Geometry: final body of the model. Coordinates: model frame, mm. Face numbers are marked on the shaded views. Round coordinates to 2 decimals unless told otherwise and drop trailing zeros. Order: outer loops, then holes, each group sorted by start corner. A loop starts at its lowest first (then second) coordinate and runs counter-clockwise, first axis right, second up. Notation, with made-up numbers: M -14,5 L -2,5 A16 cw -2,13 Z; hole C 27.5,24.5 d10. An arc over 180 degrees is marked long. Put each result on its own line as item: value. Start each with the question number.
1) Material intervals for probe 1 along X at (y, z) = (3, 5.25); probe 2 along Y at (x, z) = (42.5, 6); probe 3 along X at (y, z) = (16, 6.75), sorted ascending. Write a range as [from, to].
2) First-contact query: P1, Ø2, axis at y = -26, z = 3, coming from the -X side; P2, Ø2.5, axis at x = 0.5, y = -51, coming from the +Z side; P3, Ø2, axis at x = -36.5, z = 3.5, coming from the +Y side. Flat tips, straight axial feed; report the tip coordinate or a pass-through.
3) Section B-B, the plane y = -21. Return loops of the section in (x, z), then the cut area to 3 significant figures.
4) Section D-D, the plane y = 10. Return loops of the section in (x, z).
5) Section C-C, the plane z = 6.75. Count the separate pieces of the cut face and the enclosed holes in it, then the cut area to 3 significant figures.
6) Draft query along X for the marked faces 1, 2 and 3. Return one class per face: pulls with the +X half, pulls with the -X half, needs draft (parallel to the pull), parting line crosses it, or undercut.
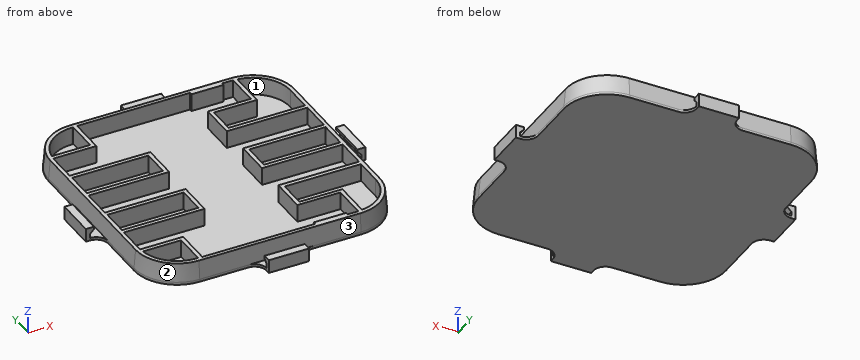
from build123d import *

# Parameters (mm, degrees)
F4_DEPTH     = 1.4
F5_W         = 30
F5_H         = 13.3
F5_W_2       = 12
F5_H_2       = 1
F6_DEPTH     = 6.6
F8_DEPTH     = 6.6
F9_W         = 14
F9_H         = 13.5
F10_DEPTH    = 6.6
F11_W        = 28.3875793553
F11_H        = 10.3
F12_DEPTH    = 6.6
F14_DEPTH    = 5.001
F15_T1_DEPTH = 1


# Not quite as in the source:
# - a fillet or chamfer that OpenCascade refuses, or shapes differently, is made with other operations: its cross-section is extruded or revolved along the edge and cut away or added


with BuildPart() as f2:
    # F2: sweep along a path in F0
    with BuildLine(Plane.XY) as f2_path:
        ThreePointArc((52, 30), (45.5563491861, 45.5563491861), (30, 52))
        Line((30, 52), (0, 52))
        Line((0, 52), (-30, 52))
        ThreePointArc((-30, 52), (-45.5563491861, 45.5563491861), (-52, 30))
        Line((-52, 30), (-52, 0))
        Line((-52, 0), (-52, -30))
        ThreePointArc((-52, -30), (-45.5563491861, -45.5563491861), (-30, -52))
        Line((-30, -52), (0, -52))
        Line((0, -52), (30, -52))
        ThreePointArc((30, -52), (45.5563491861, -45.5563491861), (52, -30))
        Line((52, -30), (52, 0))
        Line((52, 0), (52, 30))
    # F1 (on Front) → F2 (sweep)
    with BuildSketch(Plane.XZ):
        Polygon((44, 8), (44, 0), (52, 0), (52, 1), (52, 5), (49, 5), (49, 4), (50.5, 2.5), (50.5, 1), (46, 1), (45.3875793553, 8), align=None)
    sweep(path=f2_path.line)

    # F3 (on Top) → F4 (join)
    with BuildSketch(Plane.XY):
        with BuildLine():
            ThreePointArc((-44, -30), (-39.8994949366, -39.8994949366), (-30, -44))
            Line((-30, -44), (30, -44))
            ThreePointArc((30, -44), (39.8994949366, -39.8994949366), (44, -30))
            Line((44, -30), (44, 30))
            ThreePointArc((44, 30), (39.8994949366, 39.8994949366), (30, 44))
            Line((30, 44), (-30, 44))
            ThreePointArc((-30, 44), (-39.8994949366, 39.8994949366), (-44, 30))
            Line((-44, 30), (-44, -30))
        make_face()
    extrude(amount=F4_DEPTH)

    # F5 (on face) → F6 (join, through all)
    with BuildSketch(Plane.XY.offset(1.4)):
        with Locations((29, 24.85)):
            Rectangle(F5_W, F5_H)
        with Locations((20, 43.5)):
            Rectangle(F5_W_2, F5_H_2)
        with Locations((29, 0.05)):
            Rectangle(F5_W, F5_H)
        with Locations((29, -24.75)):
            Rectangle(F5_W, F5_H)
        with Locations((20, -43.5)):
            Rectangle(F5_W_2, F5_H_2)
        with BuildLine():
            ThreePointArc((-30, 44), (-39.7211110476, 40.0747208398), (-43.9910685796, 30.5))
            Line((-43.9910685796, 30.5), (-14, 30.5))
            Line((-14, 30.5), (-14, 44))
            Line((-14, 44), (-30, 44))
        make_face()
        with BuildLine():
            Line((-43.9910685796, 30.5), (-44, 30.5))
            Line((-44, 30.5), (-44, 30))
            ThreePointArc((-44, 30), (-43.9977669668, 30.250039882), (-43.9910685796, 30.5))
        make_face()
        with BuildLine():
            Line((-44, -30.5), (-43.9910685796, -30.5))
            ThreePointArc((-43.9910685796, -30.5), (-43.9977669668, -30.250039882), (-44, -30))
            Line((-44, -30), (-44, -30.5))
        make_face()
        with BuildLine():
            Line((-30, -44), (-14, -44))
            Line((-14, -44), (-14, -30.5))
            Line((-14, -30.5), (-43.9910685796, -30.5))
            ThreePointArc((-43.9910685796, -30.5), (-39.7211110476, -40.0747208398), (-30, -44))
        make_face()
        with Locations((-29, 12.35)):
            Rectangle(F5_W, F5_H)
        with Locations((-29, -12.45)):
            Rectangle(F5_W, F5_H)
    extrude(amount=F6_DEPTH)

    # F7 (on face) → F8 (join, through all)
    with BuildSketch(Plane.XY.offset(1.4)):
        with BuildLine():
            Line((43.9298241195, -31.4), (30, -31.4))
            Line((30, -31.4), (30, -44))
            ThreePointArc((30, -44), (39.3914855055, -40.3826778819), (43.9298241195, -31.4))
        make_face()
        with BuildLine():
            ThreePointArc((43.9194109071, 31.5), (39.3541434669, 40.416333328), (30, 44))
            Line((30, 44), (30, 31.5))
            Line((30, 31.5), (43.9194109071, 31.5))
        make_face()
    extrude(amount=F8_DEPTH)

    # F9 (on face) → F10 (cut, through all)
    with BuildSketch(Plane.XY.offset(8)):
        with Locations((-21, 37.25)):
            Rectangle(F9_W, F9_H)
        with Locations((-21, -37.25)):
            Rectangle(F9_W, F9_H)
    extrude(amount=-F10_DEPTH, mode=Mode.SUBTRACT)

    # F11 (on face) → F12 (cut, through all)
    with BuildSketch(Plane.XY.offset(8)):
        with BuildLine():
            Line((-43.7428112244, 32), (-29.5, 32))
            Line((-29.5, 32), (-29.5, 43.8875793553))
            Line((-29.5, 43.8875793553), (-30, 43.8875793553))
            ThreePointArc((-30, 43.8875793553), (-39.0854196832, 40.5033332581), (-43.7428112244, 32))
        make_face()
        with BuildLine():
            Line((15.5, 19.6999999465), (43.8875793553, 19.6999999465))
            Line((43.8875793553, 19.6999999465), (43.8875793553, 29.9999999465))
            ThreePointArc((43.8875793553, 30), (40.3367361721, 39.274521317), (31.5, 43.8063340663))
            Line((31.5, 43.8063340663), (31.5, 29.9999999465))
            Line((31.5, 29.9999999465), (15.5, 29.9999999465))
            Line((15.5, 29.9999999465), (15.5, 19.6999999465))
        make_face()
        with Locations((29.6937896777, 0.05)):
            Rectangle(F11_W, F11_H)
        with BuildLine():
            Line((31.5, -29.9999999465), (31.5, -43.8063340663))
            ThreePointArc((31.5, -43.8063340663), (40.3367361721, -39.274521317), (43.8875793553, -30))
            Line((43.8875793553, -29.9999999465), (43.8875793553, -29.9))
            Line((43.8875793553, -29.9), (43.8875793553, -19.6999999465))
            Line((43.8875793553, -19.6999999465), (15.5, -19.6999999465))
            Line((15.5, -19.6999999465), (15.5, -29.9))
            Line((15.5, -29.9), (15.5, -29.9999999465))
            Line((15.5, -29.9999999465), (31.5, -29.9999999465))
        make_face()
        with Locations((-29.6937896777, 12.35)):
            Rectangle(F11_W, F11_H)
        with Locations((-29.6937896777, -12.45)):
            Rectangle(F11_W, F11_H)
        with BuildLine():
            Line((-29.5, -32), (-43.7428112244, -32))
            ThreePointArc((-43.7428112244, -32), (-39.0854196832, -40.5033332581), (-30, -43.8875793553))
            Line((-30, -43.8875793553), (-29.5, -43.8875793553))
            Line((-29.5, -43.8875793553), (-29.5, -32))
        make_face()
    extrude(amount=-F12_DEPTH, mode=Mode.SUBTRACT)

    # F13 (on Top) → F14 (cut, through all)
    with BuildSketch(Plane.XY):
        with BuildLine():
            Line((52, -30), (52, -7.5))
            Line((52, -7.5), (46, -7.5))
            Line((46, -7.5), (46, -30))
            ThreePointArc((46, -30), (41.313708499, -41.313708499), (30, -46))
            Line((30, -46), (7.5, -46))
            Line((7.5, -46), (7.5, -52))
            Line((7.5, -52), (30, -52))
            ThreePointArc((30, -52), (45.5563491861, -45.5563491861), (52, -30))
        make_face()
        with BuildLine():
            Line((-30, -52), (-7.5, -52))
            Line((-7.5, -52), (-7.5, -46))
            Line((-7.5, -46), (-30, -46))
            ThreePointArc((-30, -46), (-41.313708499, -41.313708499), (-46, -30))
            Line((-46, -30), (-46, -7.5))
            Line((-46, -7.5), (-52, -7.5))
            Line((-52, -7.5), (-52, -30))
            ThreePointArc((-52, -30), (-45.5563491861, -45.5563491861), (-30, -52))
        make_face()
        with BuildLine():
            Line((-7.5, 46), (-7.5, 52))
            Line((-7.5, 52), (-30, 52))
            ThreePointArc((-30, 52), (-45.5563491861, 45.5563491861), (-52, 30))
            Line((-52, 30), (-52, 7.5))
            Line((-52, 7.5), (-46, 7.5))
            Line((-46, 7.5), (-46, 30))
            ThreePointArc((-46, 30), (-41.313708499, 41.313708499), (-30, 46))
            Line((-30, 46), (-7.5, 46))
        make_face()
        with BuildLine():
            ThreePointArc((30, 46), (41.313708499, 41.313708499), (46, 30))
            Line((46, 30), (46, 7.5))
            Line((46, 7.5), (52, 7.5))
            Line((52, 7.5), (52, 30))
            ThreePointArc((52, 30), (45.5563491861, 45.5563491861), (30, 52))
            Line((30, 52), (7.5, 52))
            Line((7.5, 52), (7.5, 46))
            Line((7.5, 46), (30, 46))
        make_face()
    extrude(amount=F14_DEPTH, mode=Mode.SUBTRACT)

    # F15: fillet of radius 4.5 on 8 edges, made by hand

    # F15_s2 → F15_t1 (join)
    with BuildSketch(Plane.XY):
        with BuildLine():
            ThreePointArc((-46, 12), (-47.3180194847, 8.8180194847), (-50.5, 7.5))
            Line((-50.5, 7.5), (-46, 7.5))
            Line((-46, 7.5), (-46, 12))
        make_face()
        with BuildLine():
            ThreePointArc((-12, 46), (-8.8180194847, 47.3180194847), (-7.5, 50.5))
            Line((-7.5, 50.5), (-7.5, 46))
            Line((-7.5, 46), (-12, 46))
        make_face()
        with BuildLine():
            ThreePointArc((12, 46), (8.8180194847, 47.3180194847), (7.5, 50.5))
            Line((7.5, 50.5), (7.5, 46))
            Line((7.5, 46), (12, 46))
        make_face()
        with BuildLine():
            ThreePointArc((12, -46), (8.8180194847, -47.3180194847), (7.5, -50.5))
            Line((7.5, -50.5), (7.5, -46))
            Line((7.5, -46), (12, -46))
        make_face()
        with BuildLine():
            ThreePointArc((-12, -46), (-8.8180194847, -47.3180194847), (-7.5, -50.5))
            Line((-7.5, -50.5), (-7.5, -46))
            Line((-7.5, -46), (-12, -46))
        make_face()
        with BuildLine():
            ThreePointArc((-46, -12), (-47.3180194847, -8.8180194847), (-50.5, -7.5))
            Line((-50.5, -7.5), (-46, -7.5))
            Line((-46, -7.5), (-46, -12))
        make_face()
        with BuildLine():
            ThreePointArc((46, -12), (47.3180194847, -8.8180194847), (50.5, -7.5))
            Line((50.5, -7.5), (46, -7.5))
            Line((46, -7.5), (46, -12))
        make_face()
        with BuildLine():
            ThreePointArc((46, 12), (47.3180194847, 8.8180194847), (50.5, 7.5))
            Line((50.5, 7.5), (46, 7.5))
            Line((46, 7.5), (46, 12))
        make_face()
    extrude(amount=F15_T1_DEPTH)


solid = f2.part
Result sheet:
1. probe 1: x = [-45.63, -44], [14, 15.5], [43.89, 45.63]
1. probe 2: y = [-39.27, -36.05], [-19.7, -18.1], [-6.6, -5.1], [5.2, 6.7], [18.2, 19.7], [36.05, 39.27]
1. probe 3: x = [-45.5, -43.89], [-15.5, -14], [44, 45.5]
2. P1: stops at x = -45.91
2. P2: stops at z = 5
2. P3: stops at y = 44.8
3. outline: M -46,0 L 46,0 L 46,1 L 45.39,8 L 43.89,8 L 43.89,1.4 L 15.5,1.4 L 15.5,8 L 14,8 L 14,1.4 L -44,1.4 L -44,8 L -45.39,8 L -46,1 Z
3. area: 162 mm2
4. outline: M -46.47,0 L 46.47,0 L 46.47,1 L 46,1 L 45.39,8 L 44,8 L 44,1.4 L -14,1.4 L -14,8 L -15.5,8 L -15.5,1.4 L -43.89,1.4 L -43.89,8 L -45.39,8 L -46,1 L -46.47,1 Z
5. separate pieces: 1
5. enclosed holes: 8
5. area: 1,150 mm2
6. face 1: undercut
6. face 2: pulls with the -X half
6. face 3: needs draft
